```python
from build123d import *

# Parameters (mm, degrees)
SKETCH_1_R          = 5
SKETCH_1_R_2        = 1.5
SKETCH_1_R_3        = 3
EXTRUDE_1_DEPTH     = 4
SKETCH_2_W          = 74.681955409
SKETCH_2_H          = 4
EXTRUDE_2_DEPTH     = 12
SKETCH_3_R          = 2.5
CUT_EXTRUDE_1_DEPTH = 109.876048253


with BuildPart() as part:
    # 草图1 → 凸台-拉伸1 (new body)
    with BuildSketch(Plane.XY):
        with BuildLine():
            Line((-49.360062144, -0.241015089), (-23.122201524, -45.686322765))
            Line((-23.122201524, -45.686322765), (-23.122201524, -49.686322765))
            Line((-23.122201524, -49.686322765), (51.559753885, -49.686322765))
            Line((51.559753885, -49.686322765), (51.559753885, -45.686322765))
            Line((51.559753885, -45.686322765), (6.651404412, 32.097220205))
            ThreePointArc((6.651404412, 32.097220205), (-37.523446513, 43.933835837), (-49.360062144, -0.241015089))
        make_face()
        with Locations((-21.354328866, 15.928102558)):
            Circle(SKETCH_1_R, mode=Mode.SUBTRACT)
        with Locations((-29.816939203, 24.632935589)):
            Circle(SKETCH_1_R_2, mode=Mode.SUBTRACT)
        with Locations((-12.649495836, 24.390712895)):
            Circle(SKETCH_1_R_2, mode=Mode.SUBTRACT)
        with Locations((-12.89171853, 7.223269528)):
            Circle(SKETCH_1_R_2, mode=Mode.SUBTRACT)
        with Locations((-30.059161896, 7.465492222)):
            Circle(SKETCH_1_R_2, mode=Mode.SUBTRACT)
        with Locations((-3.567776343, -14.879110103)):
            Circle(SKETCH_1_R_3, mode=Mode.SUBTRACT)
        with Locations((3.675910259, -27.425543331)):
            Circle(SKETCH_1_R_3, mode=Mode.SUBTRACT)
    extrude(amount=EXTRUDE_1_DEPTH)

    # 草图2 → 凸台-拉伸2 (add)
    with BuildSketch(Plane(origin=(0, 0, 0), x_dir=(-1, 0, 0), z_dir=(0, 0, -1))):
        with Locations((-14.218776181, -47.686322765)):
            Rectangle(SKETCH_2_W, SKETCH_2_H)
    extrude(amount=EXTRUDE_2_DEPTH)

    # 草图3 → 切除-拉伸1 (cut, through all)
    with BuildSketch(Plane(origin=(0, -45.686322765, 0), x_dir=(1, 0, 0), z_dir=(0, 1, 0))):
        with Locations(Location((24.21877618, 6, 0), (0, 0, 270))):
            Circle(SKETCH_3_R)
        with Locations(Location((44.21877618, 6, 0), (0, 0, 270))):
            Circle(SKETCH_3_R)
        with Locations(Location((-15.78122382, 6, 0), (0, 0, 90))):
            Circle(SKETCH_3_R)
        with Locations(Location((4.21877618, 6, 0), (0, 0, 90))):
            Circle(SKETCH_3_R)
    extrude(amount=-CUT_EXTRUDE_1_DEPTH, mode=Mode.SUBTRACT)


solid = part.part
```
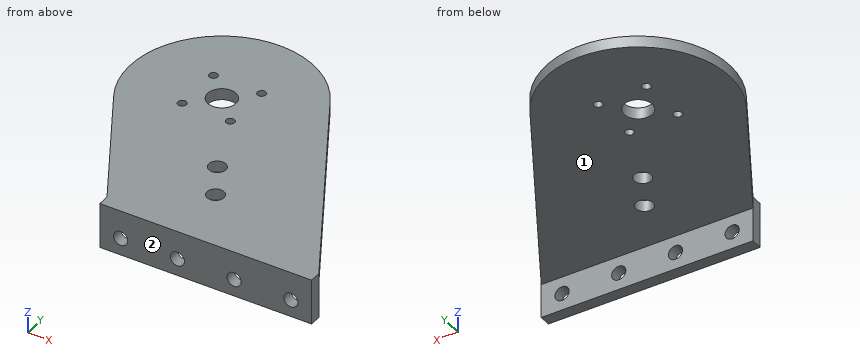
Verification items for the finished model (mm, model axes). Face numbers are marked on the shaded views. A direction names the side the tool comes from. Give positions to 0.01 mm unless a question says otherwise; leave off trailing zeros. Order: outer loops, then holes, each group sorted by start corner. A loop starts at its lowest first (then second) coordinate and runs counter-clockwise, first axis right, second up. Notation, with made-up numbers: (68.25, -20.5) -> (105.25, -20.5) arc R18 cw to (105.25, -10.5) -> close; hole circle Ø3 at (9.25, 87.5). An arc over 180 degrees is marked (long way). Use a Markdown table: item, result.
1) Material ranges on probe 1 along X at (y, z) = (-47.45, -6); probe 2 along Y at (x, z) = (16, -2.75); probe 3 along Z at (x, y) = (5.5, -9.5), recorded low to high.
Results:
| item | result |
|---|---|
| probe 1 | -23.12 to -18.28, -13.28 to 1.72, 6.72 to 21.72, 26.72 to 41.72, 46.72 to 51.56 |
| probe 2 | -49.69 to -45.69 |
| probe 3 | 0 to 4 |
2) Depth check by flat-ended pin: pin 1 Ø4.5 at (x, z) = (44.22, -6) entering from +Y; pin 2 Ø8 at (x, z) = (24.22, -6) entering from -Y; pin 3 Ø3.5 at (x, z) = (8, -6.5) entering from +Y; pin 4 Ø5 at (x, y) = (34.5, -14) entering from -Z. Enter the tip coordinate at first touch or a pass-through.
Results:
| item | result |
|---|---|
| pin 1 | through |
| pin 2 | y = -49.69 |
| pin 3 | y = -45.69 |
| pin 4 | z = 0 |
3) Section check C-C, the plane y = 18. Record the boundary of the cut face in (x, z), then the cut area to 3 significant figures.
Results:
| item | result |
|---|---|
| outline | (-53.63, 0) -> (-25.9, 0) -> (-25.9, 4) -> (-53.63, 4) -> close; (-16.8, 0) -> (14.79, 0) -> (14.79, 4) -> (-16.8, 4) -> close |
| area | 237 mm² |
4) Section check D-D, the plane z = 2.75. Record the boundary of the cut face in (x, y), then the cut area to 3 significant figures.
Results:
| item | result |
|---|---|
| outline | (-49.36, -0.24) -> (-23.12, -45.69) -> (-23.12, -49.69) -> (51.56, -49.69) -> (51.56, -45.69) -> (6.65, 32.1) arc R32.34 ccw to start; hole circle Ø3 at (-30.06, 7.47); hole circle Ø3 at (-29.82, 24.63); hole circle Ø10 at (-21.35, 15.93); hole circle Ø3 at (-12.89, 7.22); hole circle Ø3 at (-12.65, 24.39); hole circle Ø6 at (-3.57, -14.88); hole circle Ø6 at (3.68, -27.43) |
| area | 6,380 mm² |
5) Section check A-A, the plane z = -6. Record the boundary of the cut face in (x, y).
Results:
| item | result |
|---|---|
| outline | (-23.12, -49.69) -> (-18.28, -49.69) -> (-18.28, -45.69) -> (-23.12, -45.69) -> close; (-13.28, -49.69) -> (1.72, -49.69) -> (1.72, -45.69) -> (-13.28, -45.69) -> close; (6.72, -49.69) -> (21.72, -49.69) -> (21.72, -45.69) -> (6.72, -45.69) -> close; (26.72, -49.69) -> (41.72, -49.69) -> (41.72, -45.69) -> (26.72, -45.69) -> close; (46.72, -49.69) -> (51.56, -49.69) -> (51.56, -45.69) -> (46.72, -45.69) -> close |
6) Tool access check on the marked faces 1 and 2. Record the directions out of +Z, -Z, +X, -X, +Y, -Y that give a thin tool (end or side, any length) a straight path to the whole face; none if there is none.
Results:
| item | result |
|---|---|
| face 1 | -Z, +X, -X, +Y |
| face 2 | +Z, -Z, +X, -X, -Y |
7) Section check B-B, the plane x = -25. Record the boundary of the cut face in (y, z), then the cut area to 3 significant figures.
Results:
| item | result |
|---|---|
| outline | (-42.43, 0) -> (12.51, 0) -> (12.51, 4) -> (-42.43, 4) -> close; (19.35, 0) -> (48.06, 0) -> (48.06, 4) -> (19.35, 4) -> close |
| area | 335 mm² |
